Source: CAD feature listing. Evaluate the final solid. Frame: model axes, mm. A direction names the side the tool comes from. Coordinates: 2 decimals unless noted, no trailing zeros. Write each loop counter-clockwise with the first axis right and the second up, starting at its lowest first coordinate (ties: lowest second). Pieces come first, ordered by that corner, then holes. Notation, with made-up numbers: (85, 32) - (134, 32) arc R22 ccw to (134, 59) - close; hole circle Ø11 at (53, -29.5). An arc over 180 degrees is marked (long way). One line per item, written item: value.
Autodesk Inventor part; units mm, degrees
ref_plane "YZ Plane" through (0, 0, 0) normal (1, 0, 0) x (0, 1, 0)
ref_plane "XZ Plane" through (0, 0, 0) normal (0, 1, 0) x (-1, 0, 0)
ref_plane "XY Plane" through (0, 0, 0) normal (0, 0, 1) x (1, 0, 0)
sketch "Sketch2" plane through (0, 0, 0) normal (0, 1, 0) x (-1, 0, 0)
  line L0 (-47.625, 80.645) -> (47.625, 80.645)
  line L1 (47.625, 80.645) -> (47.625, -80.645)
  line L2 (47.625, -80.645) -> (-47.625, -80.645)
  line L3 (-47.625, -80.645) -> (-47.625, 80.645)
  line L4 (-47.625, 80.645) -> (47.625, -80.645) construction
  line L5 (47.625, 80.645) -> (-47.625, -80.645) construction
  point P0 (0, 0)
  dimension "d6" = 161.29
  dimension "d7" = 95.25
extrude "Extrusion2" add sketch "Sketch2" along normal blind 6.35
sketch "Sketch3" plane through (0, 6.35, 0) normal (0, 1, 0) x (1, 0, 0)
  line L0 (47.625, 80.645) -> (-47.625, 80.645)
  line L1 (47.625, -80.645) -> (-47.625, -80.645)
  line L2 (-47.625, -80.645) -> (-47.625, 80.645)
  line L3 (-47.625, 80.645) -> (47.625, 80.645)
  line L4 (47.625, 80.645) -> (47.625, -80.645)
  line L5 (47.625, -80.645) -> (-47.625, 80.645) construction
  line L6 (-47.625, -80.645) -> (47.625, 80.645) construction
  line L7 (41.275, -74.295) -> (-41.275, -74.295)
  line L8 (-41.275, -74.295) -> (-41.275, 74.295)
  line L9 (-41.275, 74.295) -> (41.275, 74.295)
  line L10 (41.275, 74.295) -> (41.275, -74.295)
  line L11 (41.275, -74.295) -> (-41.275, 74.295) construction
  line L12 (-41.275, -74.295) -> (41.275, 74.295) construction
  point P0 (0, 0)
  dimension "d10" = 148.59
  dimension "d11" = 82.55
extrude "Extrusion3" add sketch "Sketch3" along normal blind 31.75
sketch "Sketch6" plane through (0, 38.1, 0) normal (0, 1, 0) x (1, 0, 0)
  line L0 (44.45, -77.47) -> (-44.45, -77.47)
  line L1 (-44.45, -77.47) -> (-44.45, 77.47)
  line L2 (-44.45, 77.47) -> (44.45, 77.47)
  line L3 (44.45, 77.47) -> (44.45, -77.47)
  line L4 (44.45, -77.47) -> (-44.45, 77.47) construction
  line L5 (-44.45, -77.47) -> (44.45, 77.47) construction
  point P0 (0, 0)
  dimension "d29" = 154.94
  dimension "d30" = 88.9
extrude "Extrusion6" cut sketch "Sketch6" against normal blind 4.7625
sketch "Sketch9" plane through (-47.625, 0, -80.645) normal (-1, 0, 0) x (0, 0, 1)
  line L0 (161.29, 0) -> (0, 0)
  line L1 (74.8462, 0) -> (81.1962, 0)
  line L2 (81.1962, 0) -> (81.1962, 4.1295)
  line L3 (81.1962, 4.1295) -> (74.8462, 4.1295)
  line L4 (74.8462, 4.1295) -> (74.8462, 0)
  point P0 (80.645, 0)
  dimension "d57" = 6.35
extrude "Extrusion9" add sketch "Sketch9" along normal blind 25.4
sketch "Sketch10" plane through (-47.625, 0, 80.645) normal (0, 0, 1) x (1, 0, 0)
  line L0 (95.25, 0) -> (0, 0)
  line L1 (39.3541, 0) -> (45.7041, 0)
  line L2 (45.7041, 0) -> (45.7041, 3.778)
  line L3 (45.7041, 3.778) -> (39.3541, 3.778)
  line L4 (39.3541, 3.778) -> (39.3541, 0)
  point P0 (47.625, 0)
  dimension "d56" = 6.35
extrude "Extrusion10" add sketch "Sketch10" along normal blind 25.4
sketch "Sketch11" plane through (47.625, 0, 80.645) normal (1, 0, 0) x (0, 0, -1)
  line L0 (161.29, 0) -> (0, 0)
  line L1 (86.4438, 4.1295) -> (86.4438, 0)
  line L2 (80.0938, 0) -> (86.4438, 0)
  line L3 (86.4438, 0) -> (86.4438, 4.1295)
  line L4 (86.4438, 4.1295) -> (80.0938, 4.1295)
  line L5 (80.0938, 4.1295) -> (80.0938, 0)
  point P0 (80.645, 0)
  dimension "d55" = 6.35
extrude "Extrusion11" add sketch "Sketch11" along normal blind 25.4
sketch "Sketch12" plane through (47.625, 0, -80.645) normal (0, 0, -1) x (-1, 0, 0)
  line L0 (41.275, 0) -> (47.625, 0)
  line L1 (47.625, 0) -> (47.625, 3.778)
  line L2 (47.625, 3.778) -> (41.275, 3.778)
  line L3 (41.275, 3.778) -> (41.275, 0)
  dimension "d54" = 6.35
extrude "Extrusion12" add sketch "Sketch12" along normal blind 25.4
fillet "Fillet1" radius 3.175 12 edges at (47.625, 19.05, 80.645) (47.625, 19.05, -80.645) (-47.625, 19.05, -80.645) (-47.625, 19.05, 80.645) (44.45, 35.7187, -77.47) (41.275, 19.8437, -74.295) (-41.275, 19.8437, -74.295) (-44.45, 35.7187, -77.47) (-41.275, 19.8437, 74.295) (-44.45, 35.7187, 77.47) (41.275, 19.8437, 74.295) (44.45, 35.7187, 77.47)
properties part number "iceTubeClockBase"
1) Material intervals for line 1 (X direction, y = 12, z = -23) (3 decimals); line 2 (Z direction, x = -23.5, y = 12.5) (3 decimals); line 3 (X direction, y = 2, z = 64.5) (3 decimals), sorted ascending.
Values found:
line 1: -47.625 to -41.275, 41.275 to 47.625
line 2: -80.645 to -74.295, 74.295 to 80.645
line 3: -47.625 to 47.625
2) Draft query along Z for faces 1 (the flat face through (-60, 2, 0.551)), 2 (the flat face through (-60, 4.13, -3)), 3 (the flat face through (-60, 2, -5.799)), 4 (the flat face through (-1, 20, -74.295)). Return one class per face: released by +Z, released by -Z, zero draft, split by the parting line, or undercut.
Values found:
face 1: released by +Z
face 2: zero draft
face 3: released by -Z
face 4: undercut
3) Contact query for flat-ended pins moving along their axis: P1, Ø2, axis at x = -23.5, y = 5.5, coming from the +Z side (3 decimals); P2, Ø1.2, axis at x = 56, y = 1, coming from the -Z side; P3, Ø10, axis at y = 4, z = 16.5, coming from the -X side (3 decimals). Output: stop coordinate, or through.
Values found:
P1: z = 80.645
P2: z = -5.8
P3: x = -47.625
4) Reachability of faces 5 (the flat face through (-5, 3.778, 93)), 6 (the flat face through (1, 36, 77.47)), 7 (the flat face through (3, 3.778, -93)) from +Z, -Z, +X, -X, +Y, -Y: full face, straight path, thin tool, end or side. Return the list, or none.
Values found:
face 5: +Z, +X, -X, +Y
face 6: +Y
face 7: -Z, +X, -X, +Y
5) Section query A-A on y = 30.5. Output: boundary loops of the cut face in (x, z) (3 decimals), then the cut area to 3 significant figures.
Values found:
outline: (-47.625, -77.47) arc R3.175 ccw to (-44.45, -80.645) - (44.45, -80.645) arc R3.175 ccw to (47.625, -77.47) - (47.625, 77.47) arc R3.175 ccw to (44.45, 80.645) - (-44.45, 80.645) arc R3.175 ccw to (-47.625, 77.47) - close; hole (-41.275, -71.12) arc R3.175 ccw to (-38.1, -74.295) - (38.1, -74.295) arc R3.175 ccw to (41.275, -71.12) - (41.275, 71.12) arc R3.175 ccw to (38.1, 74.295) - (-38.1, 74.295) arc R3.175 ccw to (-41.275, 71.12) - close
area: 3,100 mm2
